Part model, mm, in its own coordinate system. Face numbers are marked on the shaded views. A direction names the side the tool comes from. Give positions to 0.01 mm unless a question says otherwise; leave off trailing zeros. Write each loop counter-clockwise with the first axis right and the second up, starting at its lowest first coordinate (ties: lowest second). Pieces come first, ordered by that corner, then holes.
Autodesk Inventor part; units mm, degrees
ref_plane "YZ Plane" through (0, 0, 0) normal (1, 0, 0) x (0, 1, 0)
ref_plane "XZ Plane" through (0, 0, 0) normal (0, 1, 0) x (-1, 0, 0)
ref_plane "XY Plane" through (0, 0, 0) normal (0, 0, 1) x (1, 0, 0)
sketch "Boceto1" plane through (0, 0, 0) normal (0, 0, 1) x (1, 0, 0)
  circle A0 centre (0, 0) radius 13.25
  dimension "d0" = 26.5
extrude "Extrusión1" add sketch "Boceto1" along normal blind 49
sketch "Boceto2" plane through (0, 0, 49) normal (0, 0, 1) x (1, 0, 0)
  circle A0 centre (0, 0) radius 6.5
  dimension "d3" = 13
extrude "Extrusión2" cut sketch "Boceto2" against normal blind 5
sketch "Boceto3" plane through (0, 0, 0) normal (0, 0, -1) x (-1, 0, 0)
  circle A0 centre (0, 0) radius 6.5
  dimension "d6" = 13
extrude "Extrusión3" cut sketch "Boceto3" against normal blind 5
sketch "Boceto4" plane through (0, 0, 5) normal (0, 0, -1) x (-1, 0, 0)
  point P0 (0, 0)
  point P1 (0, 0)
sketch "Boceto5" plane through (0, 0, 44) normal (0, 0, 1) x (1, 0, 0)
  circle A0 centre (0, 0) radius 6.5
properties part number "CuerpoPrincipal_filtro"
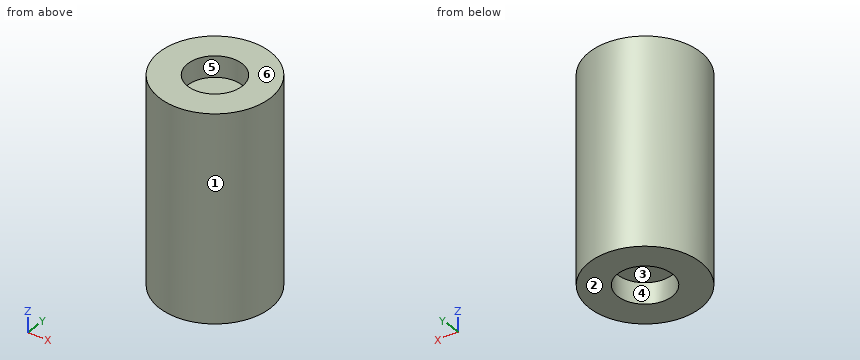
1) Mould opens along X. For the marked faces 1, 2, 3 and 4 say: +X half, -X half, draft (parallel to the pull), parting line (faces both ways), or undercut.
Check result:
face 1: parting line
face 2: draft
face 3: undercut
face 4: undercut
2) 3-axis set-ups, long thin cutter, end or side, ignore diameter. For the marked faces 5 and 6: which of +Z, -Z, +X, -X, +Y, -Y reach the whole face in a straight line?
Check result:
face 5: +Z
face 6: +Z, +X, -X, +Y, -Y
3) Saw through at B-B (x = 5.75). Write the cut outline in (y, z), and give its area (3 significant figures).
Check result:
outline: (-11.94, 0) - (-3.03, 0) - (-3.03, 5) - (3.03, 5) - (3.03, 0) - (11.94, 0) - (11.94, 49) - (3.03, 49) - (3.03, 44) - (-3.03, 44) - (-3.03, 49) - (-11.94, 49) - close
area: 1,110 mm2
4) Drill centre lines: L1, parallel to Y at x = 0, z = 3.45; L2, parallel to Z at x = -1.5, y = 0.25; L3, parallel to X at y = -3.5, z = 45.5. Where is each one in solid material? Low to high.
Check result:
L1: y = -13.25 to -6.5, 6.5 to 13.25
L2: z = 5 to 44
L3: x = -12.78 to -5.48, 5.48 to 12.78
5) Saw through at D-D (z = 9). Write the cut outline in (x, y).
Check result:
outline: circle Ø26.5 at (0, 0)
6) Saw through at A-A (z = 45.5). Write the cut outline in (x, y).
Check result:
outline: circle Ø26.5 at (0, 0); hole circle Ø13 at (0, 0)
7) Saw through at C-C (y = 0). Write the cut outline in (x, z).
Check result:
outline: (-13.25, 0) - (-6.5, 0) - (-6.5, 5) - (6.5, 5) - (6.5, 0) - (13.25, 0) - (13.25, 49) - (6.5, 49) - (6.5, 44) - (-6.5, 44) - (-6.5, 49) - (-13.25, 49) - close
8) Flat gauge pins, fed straight in: P1, Ø4, axis at x = 7.5, z = 33.5, coming from the -Y side; P2, Ø1.5, axis at y = -5, z = 28.5, coming from the -X side; P3, Ø11.5, axis at x = 0, y = 0, coming from the +Z side. Where does each tip first touch, or does it go through?
Check result:
P1: stops at y = -12.05
P2: stops at x = -12.55
P3: stops at z = 44
